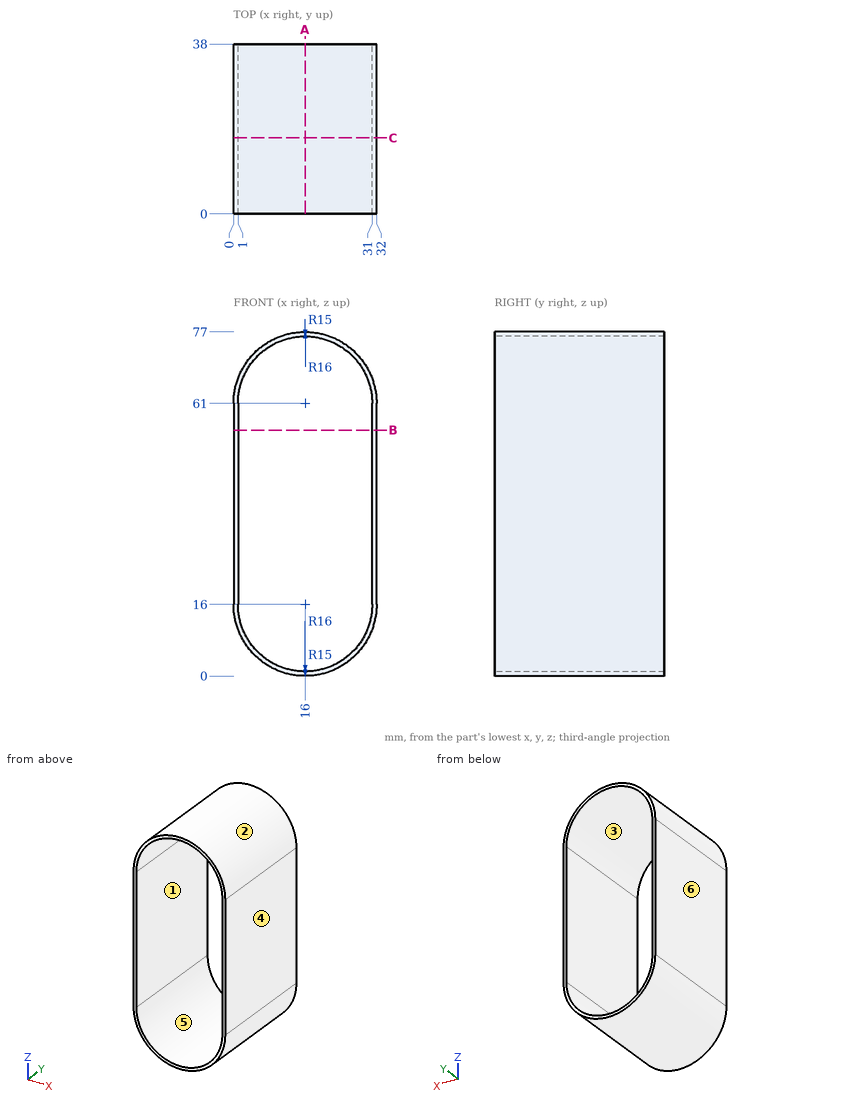
Here's the drawing with two shaded views (mm, measured from the low corner). I have some questions. A direction names the side the tool comes from. Give positions to 0.01 mm unless a question says otherwise; leave off trailing zeros. Order: outer loops, then holes, each group sorted by start corner. A loop starts at its lowest first (then second) coordinate and runs counter-clockwise, first axis right, second up. Notation, with made-up numbers: M 81.25,29.5 L 131.25,29.5 A11 cw 131.25,35.5 Z; hole C 9.25,-30 d4. An arc over 180 degrees is marked long. One line per question, with ' | ' between items.
Item 1: For the marked faces 1 and 2, which set-ups out of +Z, -Z, +X, -X, +Y, -Y let a thin tool reach every point of the face, with its end or its side?
Answer block:
face 1: +Y, -Y | face 2: +Z, +Y, -Y
Item 2: Please list where these lines run through material, in increasing order: L1, parallel to X at y = 16.5, z = 55.5; L2, parallel to Z at x = 15.5, y = 23.5; L3, parallel to X at y = 22, z = 10.
Answer block:
L1: x = 0 to 1, 31 to 32 | L2: z = 0.01 to 1.01, 75.99 to 76.99 | L3: x = 1.17 to 2.25, 29.75 to 30.83
Item 3: Suppose I cut it at A-A, the plane x = 16. Write out the boundary of the cut face in (y, z), then the cut area to 3 significant figures.
Answer block:
outline: M 0,0 L 38,0 L 38,1 L 0,1 Z; M 0,76 L 38,76 L 38,77 L 0,77 Z | area: 76.0 mm2
Item 4: I'm going to push flat-ended pins straight in: pin 1 Ø4 at (x, z) = (5, 15.5) entering from +Y; pin 2 Ø6 at (x, y) = (11.5, 12.5) entering from +Z. Where does each tip first touch, or does it pass through?
Answer block:
pin 1: passes through | pin 2: stops at z = 76.93
Item 5: Suppose I cut it at B-B, the plane z = 55. Write out the boundary of the cut face in (x, y), then the cut area to 3 significant figures.
Answer block:
outline: M 0,0 L 1,0 L 1,38 L 0,38 Z; M 31,0 L 32,0 L 32,38 L 31,38 Z | area: 76.0 mm2
Item 6: Suppose I cut it at C-C, the plane y = 17. Write out the boundary of the cut face in (x, z).
Answer block:
outline: M 0,16 A16 ccw 32,16 L 32,61 A16 ccw 0,61 Z; hole M 1,16 A15 ccw 31,16 L 31,61 A15 ccw 1,61 Z
Item 7: We'd pull the mould along X, two halves only. Please class the marked faces 3, 4, 5 and 6: released by +X, released by -X, zero draft, split by the parting line, or undercut.
Answer block:
face 3: undercut | face 4: released by +X | face 5: undercut | face 6: released by -X
